from build123d import *

# Parameters (mm, degrees)
F0_R     = 2.5
F1_DEPTH = 4


with BuildPart() as f1:
    # F0 (on Front) → F1 (new body, symmetric)
    with BuildSketch(Plane.XZ):
        with BuildLine():
            Line((-0.797178, -7.280593), (2.851209, -7.336721))
            ThreePointArc((2.851209, -7.336721), (5.361142, -6.500314), (6.8, -4.280173))
            Line((6.8, -4.280173), (6.8, 4.603175))
            ThreePointArc((6.8, 4.603175), (7.948803, 7.791949), (10.867313, 9.515414))
            Line((10.867313, 9.515414), (10.867313, 18.717312))
            ThreePointArc((10.867313, 18.717312), (10.61867, 19.366425), (10, 19.683313))
            Line((10, 19.683313), (2.86759, 19.683313))
            ThreePointArc((2.86759, 19.683313), (1.43159, 16.133334), (-2.330272, 15.417209))
            ThreePointArc((-2.330272, 15.417209), (-3.182277, 15.323191), (-3.623003, 14.587997))
            ThreePointArc((-3.623003, 14.587997), (-6.463829, 8.322883), (-8.182797, 1.66202))
            ThreePointArc((-8.182797, 1.66202), (-8.238145, 0.013758), (-8.182797, -1.634504))
            ThreePointArc((-8.182797, -1.634504), (-6.638926, -5.004085), (-8.524801, -8.194867))
            ThreePointArc((-8.524801, -8.194867), (-6.774749, -9.262294), (-4.822111, -9.88622))
            ThreePointArc((-4.822111, -9.88622), (-4.136805, -8.380333), (-2.900719, -7.280593))
            Line((-2.900719, -7.280593), (-0.797178, -7.280593))
        make_face()
        Circle(F0_R, mode=Mode.SUBTRACT)
    extrude(amount=F1_DEPTH, both=True)


solid = f1.part
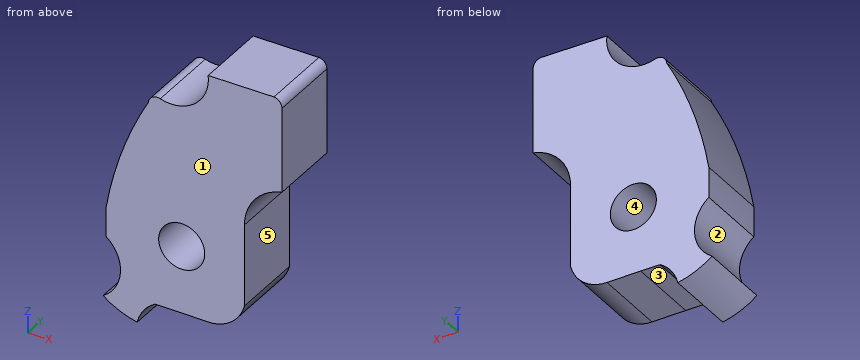
Check sheet for the modelled part. Datum: model origin and axes. Units: mm. Face numbers are marked on the shaded views. A direction names the side the tool comes from. Round coordinates to 2 decimals unless told otherwise and drop trailing zeros. Write each loop counter-clockwise with the first axis right and the second up, starting at its lowest first coordinate (ties: lowest second). Pieces come first, ordered by that corner, then holes. Notation, with made-up numbers: (11.5, -29.75) - (36.5, -29.75) arc R26 ccw to (36.5, -5.75) - close; hole circle Ø7 at (64.5, 33). An arc over 180 degrees is marked (long way). Return JSON: item names as keys, results as strings.
Q1. Scan lines: L1, parallel to Z at x = 0, y = 2; L2, parallel to X at y = 1, z = 1.5; L3, parallel to Z at x = 0.25, y = 1. Record each from-to range of solid material in increasing order. Write a range as from..to.
Returned:
{"L1": "z = -7.29..-2.5, 2.5..15.38", "L2": "x = -8.19..-2, 2..6.8", "L3": "z = -7.3..-2.49, 2.49..15.46"}
Q2. Cross-section at D-D (x = 8.25). Record the boundary of the cut face in (y, z).
Returned:
{"outline": "(-4, 8.12) - (4, 8.12) - (4, 19.68) - (-4, 19.68) - close"}
Q3. Cross-section at B-B (x = 0). Record the boundary of the cut face in (y, z).
Returned:
{"outline": "(-4, -7.29) - (4, -7.29) - (4, -2.5) - (-4, -2.5) - close; (-4, 2.5) - (4, 2.5) - (4, 15.38) - (-4, 15.38) - close"}
Q4. Cross-section at C-C (y = 3.5). Record the boundary of the cut face in (x, z), then the cut area to 3 significant figures.
Returned:
{"outline": "(-8.52, -8.19) arc R8.62 ccw to (-4.82, -9.89) arc R4 cw to (-2.9, -7.28) - (-0.8, -7.28) - (2.85, -7.34) arc R4 ccw to (6.8, -4.28) - (6.8, 4.6) arc R5 cw to (10.87, 9.52) - (10.87, 18.72) arc R0.97 ccw to (10, 19.68) - (2.87, 19.68) arc R4 cw to (-2.33, 15.42) arc R0.96 ccw to (-3.62, 14.59) arc R39.78 ccw to (-8.18, 1.66) arc R24.57 ccw to (-8.18, -1.63) arc R4 cw to start; hole circle Ø5 at (0, 0)", "area": "357 mm²"}
Q5. Depth check by flat-ended pin: P1, Ø1.1, axis at x = -2, y = -1.5, coming from the -Z side; P2, Ø2, axis at x = 5.5, y = 0, coming from the -Z side; P3, Ø2.5, axis at y = -1, z = -1.5, coming from the +X side. Enter the tip coordinate at first touch or a pass-through.
Returned:
{"P1": "stops at z = -7.28", "P2": "stops at z = -7.01", "P3": "stops at x = 6.8"}
Q6. Cross-section at A-A (z = 0). Record the boundary of the cut face in (x, y).
Returned:
{"outline": "(-8.24, -4) - (-2.5, -4) - (-2.5, 4) - (-8.24, 4) - close; (2.5, -4) - (6.8, -4) - (6.8, 4) - (2.5, 4) - close"}
Q7. Access from +Z, -Z, +X, -X, +Y, -Y to the whole of each face (thin tool, end or side, straight path). Record for the marked faces 4 and 5.
Returned:
{"face 4": "+Y, -Y", "face 5": "-Z, +X, +Y, -Y"}
Q8. Draft check along Z on the marked faces 1, 2 and 3. Enter one of: released by +Z, released by -Z, zero draft, split by the parting line, or undercut.
Returned:
{"face 1": "zero draft", "face 2": "undercut", "face 3": "released by -Z"}
